Verification items for the finished model (mm, model axes). Give positions to 0.01 mm unless a question says otherwise; leave off trailing zeros. Loops run counter-clockwise (first coordinate to the right, second up) from the corner with the lowest first, then second, coordinate; pieces in that order, holes last. Notation, with made-up numbers: (-36, 34.25) -> (-9, 34.25) arc R18 cw to (-9, 64.25) -> close; hole circle Ø10 at (89.25, -26). An arc over 180 degrees is marked (long way). Answer in a Markdown table with one row per item. Add a question column.
Q1. Section check B-B on x = 258. Enter the section's corners in (y, z), and give its area (3 significant figures).
Q2. Section check A-A on z = 4.45. Give the number of separate pieces and of enclosed holes in the cut face, and give its area (3 significant figures).
Q3. Material ranges on probe 1 along Y at (x, z) = (162, 3.2); probe 2 along X at (y, z) = (-20.5, 2.7); probe 3 along X at (y, z) = (-17.5, 1.2), recorded low to high.
```python
from build123d import *

# Parameters (mm, degrees)
SKETCH2_W           = 360
SKETCH2_H           = 40
SKETCH2_W_2         = 30
SKETCH2_H_2         = 5.54
BOSS_EXTRUDE1_DEPTH = 5.54
FILLET1_R           = 10


with BuildPart() as part:
    # Sketch2 → Boss-Extrude1 (new body)
    with BuildSketch(Plane.XY):
        with Locations((239.474602118, -4.853960239)):
            Rectangle(SKETCH2_W, SKETCH2_H)
        with Locations((89.474602118, 7.646039761)):
            Rectangle(SKETCH2_W_2, SKETCH2_H_2, mode=Mode.SUBTRACT)
        with Locations((149.474602118, 7.646039761)):
            Rectangle(SKETCH2_W_2, SKETCH2_H_2, mode=Mode.SUBTRACT)
        with Locations((209.474602118, 7.646039761)):
            Rectangle(SKETCH2_W_2, SKETCH2_H_2, mode=Mode.SUBTRACT)
        with Locations((269.474602118, 7.646039761)):
            Rectangle(SKETCH2_W_2, SKETCH2_H_2, mode=Mode.SUBTRACT)
        with Locations((329.474602118, 7.646039761)):
            Rectangle(SKETCH2_W_2, SKETCH2_H_2, mode=Mode.SUBTRACT)
        with Locations((389.474602118, 7.646039761)):
            Rectangle(SKETCH2_W_2, SKETCH2_H_2, mode=Mode.SUBTRACT)
    extrude(amount=BOSS_EXTRUDE1_DEPTH)

    # Fillet1
    fillet1_edges = [part.edges().sort_by_distance(p)[0] for p in [
        (419.474602118, -24.853960239, 2.77),
        (59.474602118, -24.853960239, 2.77),
    ]]
    fillet(fillet1_edges, radius=FILLET1_R)


solid = part.part
```
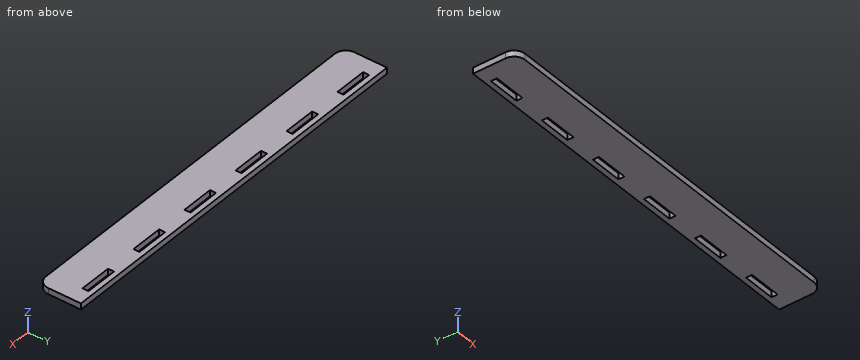
Taken from the geometry:
| question | item | result |
|---|---|---|
| 1 | outline | (-24.85, 0) -> (4.88, 0) -> (4.88, 5.54) -> (-24.85, 5.54) -> close; (10.42, 0) -> (15.15, 0) -> (15.15, 5.54) -> (10.42, 5.54) -> close |
| 1 | area | 191 mm² |
| 2 | separate pieces | 1 |
| 2 | enclosed holes | 6 |
| 2 | area | 13,400 mm² |
| 3 | probe 1 | y = -24.85 to 4.88, 10.42 to 15.15 |
| 3 | probe 2 | x = 61.22 to 417.73 |
| 3 | probe 3 | x = 59.83 to 419.12 |
